```python
from build123d import *

# Parameters (mm, degrees)
SKIZZE3_W                       = 58
SKIZZE3_H                       = 58
AUFSATZ_LINEAR_AUSTRAGEN1_DEPTH = 15
SKIZZE4_R                       = 7.5
AUFSATZ_LINEAR_AUSTRAGEN2_DEPTH = 2
FASE1_SIZE                      = 5
SKIZZE5_R                       = 23
SKIZZE5_R_2                     = 20.5
AUFSATZ_LINEAR_AUSTRAGEN3_DEPTH = 30
SKIZZE6_W                       = 3
SKIZZE6_H                       = 39.520504732
SCHNITT_LINEAR_AUSTRAGEN1_DEPTH = 6
SKIZZE7_W                       = 3
SKIZZE7_H                       = 35.12933754
SCHNITT_LINEAR_AUSTRAGEN2_DEPTH = 6
SCHNITT_LINEAR_AUSTRAGEN3_DEPTH = 53
FASE2_SIZE                      = 0.5
FASE3_SIZE                      = 0.5
SKIZZE10_W                      = 58.775237502
SKIZZE10_H                      = 7.5
SCHNITT_LINEAR_AUSTRAGEN5_DEPTH = 17


with BuildPart() as part:
    # Skizze3 → Aufsatz-Linear austragen1 (new body)
    with BuildSketch(Plane.XY):
        Rectangle(SKIZZE3_W, SKIZZE3_H)
    extrude(amount=AUFSATZ_LINEAR_AUSTRAGEN1_DEPTH)

    # Skizze4 → Aufsatz-Linear austragen2 (add)
    with BuildSketch(Plane(origin=(0, 0, 0), x_dir=(-1, 0, 0), z_dir=(0, 0, -1))):
        with Locations(Location((0, 19, 0), (0, 0, 180))):  # turned: the seam where the file's is
            Circle(SKIZZE4_R)
        with Locations(Location((19, -19, 0), (0, 0, 180))):  # turned: the seam where the file's is
            Circle(SKIZZE4_R)
        with Locations(Location((-19, -19, 0), (0, 0, 180))):  # turned: the seam where the file's is
            Circle(SKIZZE4_R)
    extrude(amount=AUFSATZ_LINEAR_AUSTRAGEN2_DEPTH)

    # Fase1
    fase1_edges = [part.edges().sort_by_distance(p)[0] for p in [
        (29, -29, 7.5),
        (-29, -29, 7.5),
        (-29, 29, 7.5),
        (29, 29, 7.5),
    ]]
    chamfer(fase1_edges, length=FASE1_SIZE)

    # Skizze5 → Aufsatz-Linear austragen3 (add)
    with BuildSketch(Plane.XY.offset(15)):
        Circle(SKIZZE5_R)
        Circle(SKIZZE5_R_2, mode=Mode.SUBTRACT)
    extrude(amount=AUFSATZ_LINEAR_AUSTRAGEN3_DEPTH)

    # Skizze6 → Schnitt-Linear austragen1 (cut)
    with BuildSketch(Plane(origin=(0, -23, 0), x_dir=(0, 0, -1), z_dir=(0, -1, 0))):
        with Locations((-23.5, 0)):
            Rectangle(SKIZZE6_W, SKIZZE6_H)
        with Locations((-31, 0)):
            Rectangle(SKIZZE6_W, SKIZZE6_H)
        with Locations((-38.5, 0)):
            Rectangle(SKIZZE6_W, SKIZZE6_H)
    extrude(amount=-SCHNITT_LINEAR_AUSTRAGEN1_DEPTH, mode=Mode.SUBTRACT)

    # Skizze7 → Schnitt-Linear austragen2 (cut)
    with BuildSketch(Plane(origin=(0, 23, 0), x_dir=(0, 0, -1), z_dir=(0, 1, 0))):
        with Locations((-23.5, 0)):
            Rectangle(SKIZZE7_W, SKIZZE7_H)
        with Locations((-31, 0)):
            Rectangle(SKIZZE7_W, SKIZZE7_H)
        with Locations((-38.5, 0)):
            Rectangle(SKIZZE7_W, SKIZZE7_H)
    extrude(amount=-SCHNITT_LINEAR_AUSTRAGEN2_DEPTH, mode=Mode.SUBTRACT)

    # Skizze8 → Schnitt-Linear austragen3 (cut, through all)
    with BuildSketch(Plane(origin=(23, 0, 0), x_dir=(0, 0, -1), z_dir=(1, 0, 0))):
        with BuildLine():
            Line((-37.5, 2.5), (-22.5, 2.5))
            ThreePointArc((-22.5, 2.5), (-20, 0), (-22.5, -2.5))
            Line((-22.5, -2.5), (-37.5, -2.5))
            ThreePointArc((-37.5, -2.5), (-40, 0), (-37.5, 2.5))
        make_face()
    extrude(amount=-SCHNITT_LINEAR_AUSTRAGEN3_DEPTH, mode=Mode.SUBTRACT)

    # Fase2
    fase2_edges = [part.edges().sort_by_distance(p)[0] for p in [
        (-7.5, 19, -2),
        (-26.5, -19, -2),
        (11.5, -19, -2),
        (-23, 0, 45),
        (-20.5, 0, 45),
    ]]
    chamfer(fase2_edges, length=FASE2_SIZE)

    # Fase3
    fase3_edges = [part.edges().sort_by_distance(p)[0] for p in [
        (0, -29, 0),
        (0, -29, 15),
        (29, 0, 0),
        (-29, 0, 0),
        (0, 29, 0),
        (-26.5, 26.5, 0),
        (26.5, 26.5, 0),
        (26.5, -26.5, 0),
        (-26.5, -26.5, 0),
        (-29, 0, 15),
        (29, 0, 15),
        (0, 29, 15),
        (-26.5, 26.5, 15),
        (26.5, 26.5, 15),
        (26.5, -26.5, 15),
        (-26.5, -26.5, 15),
    ]]
    chamfer(fase3_edges, length=FASE3_SIZE)

    # Skizze10 → Schnitt-Linear austragen5 (cut)
    with BuildSketch(Plane.XZ.offset(29)):
        with Locations((0, 7.5)):
            Rectangle(SKIZZE10_W, SKIZZE10_H)
    extrude(amount=-SCHNITT_LINEAR_AUSTRAGEN5_DEPTH, mode=Mode.SUBTRACT)


solid = part.part
```
The model under review builds one solid part; all positions refer to its coordinate system, in mm. A direction names the side the tool comes from. Round coordinates to 2 decimals unless told otherwise and drop trailing zeros. Loops run counter-clockwise (first coordinate to the right, second up) from the corner with the lowest first, then second, coordinate; pieces in that order, holes last.
Item 1: For line 1 (Y direction, x = 0, z = 25.75); line 2 (Z direction, x = -21.5, y = -12.5); line 3 (Z direction, x = -13.5, y = -25), list the stretches that pass through material, from the lowest coordinate up.
Determined:
line 1: y = -23 to -20.5, 20.5 to 23
line 2: z = -2 to 3.75, 11.25 to 15
line 3: z = 0 to 3.75, 11.25 to 15
Item 2: Clearance check with flat-ended pins moving along their axes: pin 1 Ø2 at (x, z) = (-21.5, 31.5) entering from +Y; pin 2 Ø6 at (x, z) = (19.5, 33.5) entering from -Y; pin 3 Ø2.5 at (x, z) = (13, 38) entering from +Y. State where each tip first meets the part, or that it passes through.
Determined:
pin 1: stops at y = 10.43
pin 2: stops at y = -16.02
pin 3: stops at y = 19.47
Item 3: For faces 1 (the face through (0, 21, 37)), 2 (the face through (-22, 0, 40)), 3 (the face through (0, -21, 25)), list the 3-axis set-ups (+Z, -Z, +X, -X, +Y, -Y) from which the entire face can be reached by the end or side of a thin tool; tool diameter is ignored.
Determined:
face 1: +X, -X, +Y
face 2: +X, -X
face 3: +X, -X, -Y
Item 4: Take a section at D-D (z = 5). Write out the cut boundary in (x, y).
Determined:
outline: (-29, -12) - (29, -12) - (29, 24) - (24, 29) - (-24, 29) - (-29, 24) - close
Item 5: Take a section at C-C (x = 0). Give the number of separate pieces and of enclosed holes in the cut face, then the cut area to 3 significant figures.
Determined:
separate pieces: 7
enclosed holes: 0
area: 876 mm2
Item 6: Take a section at A-A (y = 0). Write out the cut boundary in (x, z).
Determined:
outline: (-29, 0.5) - (-28.5, 0) - (28.5, 0) - (29, 0.5) - (29, 14.5) - (28.5, 15) - (23, 15) - (23, 20) - (20.5, 20) - (20.5, 15) - (-20.5, 15) - (-20.5, 20) - (-23, 20) - (-23, 15) - (-28.5, 15) - (-29, 14.5) - close; (-23, 40) - (-20.5, 40) - (-20.5, 44.5) - (-21, 45) - (-22.5, 45) - (-23, 44.5) - close; (20.5, 40) - (23, 40) - (23, 44.5) - (22.5, 45) - (21, 45) - (20.5, 44.5) - close
Item 7: Mouldability with a two-part tool opening along Y and no side actions: class faces 4 (the face through (-26.36, -26.29, 14.75)), 5 (the face through (22, -2.5, 30)), 6 (the face through (21.938, 6.909, 29.544)), 7 (the face through (0, 21, 40)) as released by +Y, released by -Y, zero draft, split by the parting line, or undercut.
Determined:
face 4: released by -Y
face 5: undercut
face 6: split by the parting line
face 7: zero draft
